Verification items for the finished model (mm, model axes). Face numbers are marked on the shaded views. A direction names the side the tool comes from. Give positions to 0.01 mm unless a question says otherwise; leave off trailing zeros. Loops run counter-clockwise (first coordinate to the right, second up) from the corner with the lowest first, then second, coordinate; pieces in that order, holes last. Notation, with made-up numbers: (-38.75, -2.75) - (17.25, -2.75) arc R14 cw to (17.25, 3.25) - close; hole circle Ø3 at (62, -37). An arc over 180 degrees is marked (long way). Answer in a Markdown table with one row per item.
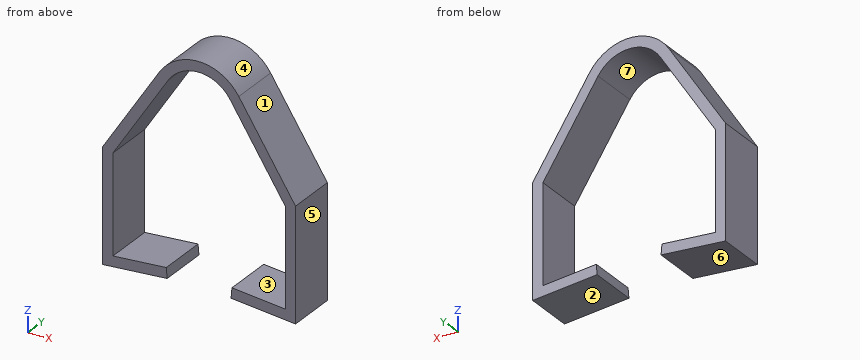
```python
from build123d import *

# Parameters (mm, degrees)
F1_DEPTH = 19.05


with BuildPart() as f1:
    # F0 (on Front) → F1 (new body)
    with BuildSketch(Plane.XZ):
        with BuildLine():
            ThreePointArc((-12.014405, 7.732188), (0, 14.2875), (12.014405, 7.732188))
            Line((12.014405, 7.732188), (33.3375, -25.4))
            Line((33.3375, -25.4), (33.3375, -63.5))
            Line((33.3375, -63.5), (12.7, -61.694453))
            Line((12.7, -61.694453), (12.354654, -65.641775))
            Line((12.354654, -65.641775), (37.2999, -67.824201))
            Line((37.2999, -67.824201), (37.2999, -24.235141))
            Line((37.2999, -24.235141), (15.3464, 9.876581))
            ThreePointArc((15.3464, 9.876581), (0, 18.2499), (-15.3464, 9.876581))
            Line((-15.3464, 9.876581), (-37.2999, -24.235141))
            Line((-37.2999, -24.235141), (-37.2999, -67.824201))
            Line((-37.2999, -67.824201), (-12.354654, -65.641775))
            Line((-12.354654, -65.641775), (-12.7, -61.694453))
            Line((-12.7, -61.694453), (-33.3375, -63.5))
            Line((-33.3375, -63.5), (-33.3375, -25.4))
            Line((-33.3375, -25.4), (-12.014405, 7.732188))
        make_face()
    extrude(amount=F1_DEPTH)


solid = f1.part
```
Q1. Thickness scan on line 1 (X direction, y = -11, z = -27); line 2 (X direction, y = -13.75, z = -23.5); line 3 (Z direction, x = 32.5, y = -14.5). Record the ranges inside material, lowest first.
Completed:
| item | result |
|---|---|
| line 1 | -37.3 to -33.34, 33.34 to 37.3 |
| line 2 | -36.83 to -32.11, 32.11 to 36.83 |
| line 3 | -67.4 to -63.43, -24.1 to -16.78 |
Q2. Sectioned sample at B-B (x = 25). Record the cut outline in (y, z).
Completed:
| item | result |
|---|---|
| outline | (-19.05, -66.75) - (0, -66.75) - (0, -62.77) - (-19.05, -62.77) - close; (-19.05, -12.45) - (0, -12.45) - (0, -5.12) - (-19.05, -5.12) - close |
Q3. Draft check along X on the marked faces 4, 5, 6 and 7. Enter one of: +X half, -X half, draft (parallel to the pull), parting line (faces both ways), or undercut.
Completed:
| item | result |
|---|---|
| face 4 | parting line |
| face 5 | +X half |
| face 6 | undercut |
| face 7 | undercut |
Q4. Sectioned sample at A-A (z = -27). Record the cut outline in (x, y).
Completed:
| item | result |
|---|---|
| outline | (-37.3, -19.05) - (-33.34, -19.05) - (-33.34, 0) - (-37.3, 0) - close; (33.34, -19.05) - (37.3, -19.05) - (37.3, 0) - (33.34, 0) - close |
Q5. Tool access check on the marked faces 1, 2 and 3. Record the directions out of +Z, -Z, +X, -X, +Y, -Y that give a thin tool (end or side, any length) a straight path to the whole face; none if there is none.
Completed:
| item | result |
|---|---|
| face 1 | +Z, +X, +Y, -Y |
| face 2 | -Z, +Y, -Y |
| face 3 | +Y, -Y |
Q6. Sectioned sample at D-D (x = -5). Record the cut outline in (y, z).
Completed:
| item | result |
|---|---|
| outline | (-19.05, 13.38) - (0, 13.38) - (0, 17.55) - (-19.05, 17.55) - close |
Q7. Go/stop test with flat-tipped pins: P1, Ø6, axis at x = -26, y = -11.5, coming from the -Z side; P2, Ø4, axis at y = -3.5, z = 3, coming from the +X side; P3, Ø6, axis at x = 2, y = -5.5, coming from the +Z side. Record where each tip stops, or that it passes through.
Completed:
| item | result |
|---|---|
| P1 | z = -67.1 |
| P2 | x = 21.06 |
| P3 | z = 18.25 |
Q8. Sectioned sample at C-C (y = -12.5). Record the cut outline in (x, z) (1 decimal), and give its area (3 significant figures).
Completed:
| item | result |
|---|---|
| outline | (-37.3, -67.8) - (-12.4, -65.6) - (-12.7, -61.7) - (-33.3, -63.5) - (-33.3, -25.4) - (-12, 7.7) arc R14.3 cw to (12, 7.7) - (33.3, -25.4) - (33.3, -63.5) - (12.7, -61.7) - (12.4, -65.6) - (37.3, -67.8) - (37.3, -24.2) - (15.3, 9.9) arc R18.2 ccw to (-15.3, 9.9) - (-37.3, -24.2) - close |
| area | 951 mm^2 |
